from build123d import *

# Parameters (mm, degrees)
SKETCH_1_W      = 115
SKETCH_1_H      = 115
SKETCH_1_R      = 7.5
EXTRUDE_1_DEPTH = 5


with BuildPart() as part:
    # 草圖1 → 填料-伸長1 (new body)
    with BuildSketch(Plane(origin=(0, 0, 0), x_dir=(0, 0, -1), z_dir=(1, 0, 0))):
        with Locations((19.013157895, 51.611842105)):
            Rectangle(SKETCH_1_W, SKETCH_1_H)
        with Locations((-23.486842105, 49.111842105)):
            Circle(SKETCH_1_R, mode=Mode.SUBTRACT)
    extrude(amount=-EXTRUDE_1_DEPTH)


solid = part.part
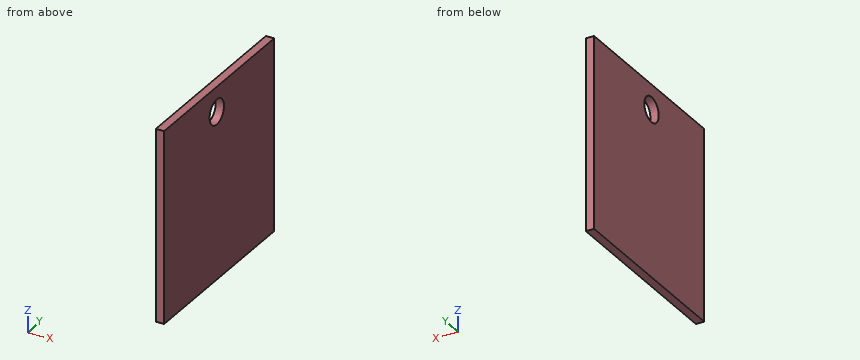
Could you check a few things on this model? Use its own coordinates, in mm. Give positions to 0.01 mm unless a question says otherwise; leave off trailing zeros. Write each loop counter-clockwise with the first axis right and the second up, starting at its lowest first coordinate (ties: lowest second). Pieces come first, ordered by that corner, then holes. Notation, with made-up numbers: (29.5, -14) -> (47.5, -14) arc R17 cw to (47.5, 0) -> close; hole circle Ø9 at (-5, -27). An arc over 180 degrees is marked (long way). Write each question's results on one line, items separated by ' | '. Start each with the question number.
Q1. I need wall thicknesses on probe 1 along Z at (x, y) = (-0.6, 56); probe 2 along Y at (x, z) = (-3.3, 26.5); probe 3 along Z at (x, y) = (-1, 45.5). Which ranges of each line are inside material? Lowest first, please.
Q2. Suppose I cut it at A-A, the plane z = 26. List the corners of the cut face in (x, y) for me, and give its area (3 significant figures).
Q3. Suppose I cut it at B-B, the plane y = 44. List the corners of the cut face in (x, z) for me, and give its area (3 significant figures).
Outcome:
1) probe 1: -76.51 to 20.52, 26.45 to 38.49 | probe 2: -5.89 to 42.24, 55.98 to 109.11 | probe 3: -76.51 to 16.91, 30.06 to 38.49
2) outline: (-5, -5.89) -> (0, -5.89) -> (0, 42.05) -> (-5, 42.05) -> close; (-5, 56.18) -> (0, 56.18) -> (0, 109.11) -> (-5, 109.11) -> close | area: 504 mm2
3) outline: (-5, -76.51) -> (0, -76.51) -> (0, 18) -> (-5, 18) -> close; (-5, 28.97) -> (0, 28.97) -> (0, 38.49) -> (-5, 38.49) -> close | area: 520 mm2
